Check sheet for the modelled part. Datum: model origin and axes. Units: mm. Coordinates: 2 decimals unless noted, no trailing zeros. Write each loop counter-clockwise with the first axis right and the second up, starting at its lowest first coordinate (ties: lowest second). Pieces come first, ordered by that corner, then holes. Notation, with made-up numbers: (-35.75, -16.75) - (-8.75, -16.75) arc R15 ccw to (-8.75, 6.25) - close; hole circle Ø2 at (-0.5, 68). An arc over 180 degrees is marked (long way). Use one line per item in the form item = value. Start each with the question number.
1. Cross-section at B-B on x = 5. Record the boundary of the cut face in (y, z).
2. Cross-section at A-A on y = 1.2. Give the number of separate pieces and of enclosed holes in the cut face, then the cut area to 3 significant figures.
3. Draft check along X on faces 1 (the face through (99, 3, 0)), 2 (the face through (133.336, 3.042, -5.026)), 3 (the face through (200, 3, -4)). Enter one of: +X half, -X half, draft (parallel to the pull), parting line (faces both ways), or undercut.
4. Go/stop test with a flat-tipped pin: pin 1 Ø2 at (x, z) = (5, -4.5) entering from -Y. Record where the tip stops, or that it passes through.
5. Scan line: line 1 along Z through (x, y) = (5, 3.25). Record every from-to range of solid material in increasing order.
```python
from build123d import *

# Parameters (mm, degrees)
SKETCH1_W           = 200
SKETCH1_H           = 9
BOSS_EXTRUDE1_DEPTH = 6
SKETCH2_R           = 1.75
CUT_EXTRUDE1_DEPTH  = 6
LPATTERN1_COUNT     = 10
LPATTERN1_PITCH     = 21.111111111


with BuildPart() as part:
    # Sketch1 → Boss-Extrude1 (new body)
    with BuildSketch(Plane(origin=(0, 0, 0), x_dir=(1, 0, 0), z_dir=(0, 1, 0))):
        with Locations((100, 4.5)):
            Rectangle(SKETCH1_W, SKETCH1_H)
    extrude(amount=BOSS_EXTRUDE1_DEPTH)

    # Sketch2 → Cut-Extrude1 (cut)
    with BuildSketch(Plane(origin=(0, 6, 0), x_dir=(1, 0, 0), z_dir=(0, 1, 0))):
        with Locations((5, 4.5)):
            Circle(SKETCH2_R)
    cut_extrude1 = extrude(amount=-CUT_EXTRUDE1_DEPTH, mode=Mode.SUBTRACT)

    # LPattern1: Cut-Extrude1 ×10
    with Locations(*[(i * LPATTERN1_PITCH, 0, 0) for i in range(1, LPATTERN1_COUNT)]):
        add(cut_extrude1, mode=Mode.SUBTRACT)


solid = part.part
```
Final values:
q1.outline = (0, -9) - (6, -9) - (6, -6.25) - (0, -6.25) - close; (0, -2.75) - (6, -2.75) - (6, 0) - (0, 0) - close
q2.separate_pieces = 1
q2.enclosed_holes = 10
q2.area = 1,700 mm²
q3.face_1 = draft
q3.face_2 = undercut
q3.face_3 = +X half
q4.pin_1 = through
q5.line_1 = -9 to -6.25, -2.75 to 0
